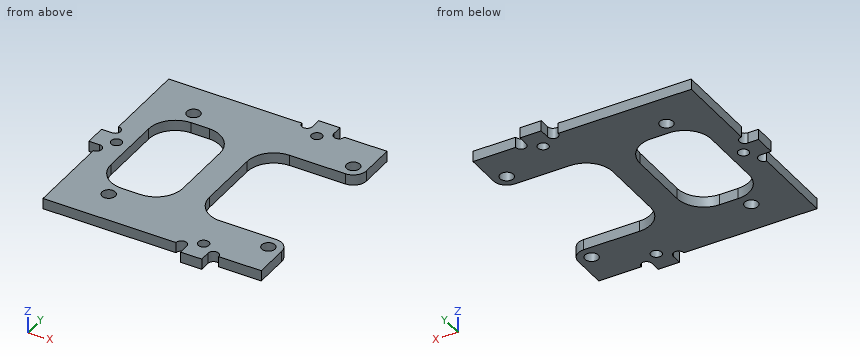
from build123d import *

# Parameters (mm, degrees)
SKETCH_1_R          = 1.25
SKETCH_1_R_2        = 1
EXTRUDE_1_DEPTH     = 2
SKETCH_4_W          = 18
SKETCH_4_H          = 22
CUT_EXTRUDE_1_DEPTH = 2
FILLET_2_R          = 2.5
FILLET_3_R          = 5
CUT_EXTRUDE_2_DEPTH = 2
SKETCH_7_R          = 1
CUT_EXTRUDE_3_DEPTH = 10
SKETCH_8_W          = 4
SKETCH_8_H          = 2
EXTRUDE_2_DEPTH     = 2
CUT_EXTRUDE_4_DEPTH = 2


with BuildPart() as part:
    # 草圖1 → 填料-伸長1 (new body)
    with BuildSketch(Plane.XY):
        Polygon((15.283786802, 18.1625), (-25.716213198, 18.1625), (-25.716213198, 0.1625), (-27.716213198, 0.1625), (-27.716213198, -3.8375), (-25.716213198, -3.8375), (-25.716213198, -21.8375), (15.283786802, -21.8375), align=None)
        with Locations((-17.216213198, 11.6625)):
            Circle(SKETCH_1_R, mode=Mode.SUBTRACT)
        with Locations((-17.216213198, -15.3375)):
            Circle(SKETCH_1_R, mode=Mode.SUBTRACT)
        with Locations((12.783786802, -15.3375)):
            Circle(SKETCH_1_R, mode=Mode.SUBTRACT)
        with Locations((12.783786802, 11.6625)):
            Circle(SKETCH_1_R, mode=Mode.SUBTRACT)
        with Locations((-23.716213198, -1.8375)):
            Circle(SKETCH_1_R_2, mode=Mode.SUBTRACT)
    extrude(amount=EXTRUDE_1_DEPTH)

    # 草圖4 → 除料-伸長1 (cut)
    with BuildSketch(Plane(origin=(0, 0, 0), x_dir=(-1, 0, 0), z_dir=(0, 0, -1))):
        with Locations((-6.283786802, -1.8375)):
            Rectangle(SKETCH_4_W, SKETCH_4_H)
    extrude(amount=-CUT_EXTRUDE_1_DEPTH, mode=Mode.SUBTRACT)

    # 圓角2
    fillet_2_edges = [part.edges().sort_by_distance(p)[0] for p in [
        (15.283786802, -12.8375, 1),
        (15.283786802, 9.1625, 1),
    ]]
    fillet(fillet_2_edges, radius=FILLET_2_R)

    # 圓角3
    fillet_3_edges = [part.edges().sort_by_distance(p)[0] for p in [
        (-2.716213198, 9.1625, 1),
        (-2.716213198, -12.8375, 1),
    ]]
    fillet(fillet_3_edges, radius=FILLET_3_R)

    # 草圖5 → 除料-伸長2 (cut)
    with BuildSketch(Plane(origin=(0, 0, 0), x_dir=(-1, 0, 0), z_dir=(0, 0, -1))):
        with BuildLine():
            Line((7.716213198, 3.948031945), (7.716213198, -7.8375))
            ThreePointArc((7.716213198, -7.8375), (9.180679292, -11.373033906), (12.716213198, -12.8375))
            Line((12.716213198, -12.8375), (16.216213198, -12.8375))
            ThreePointArc((16.216213198, -12.8375), (19.751747104, -11.373033906), (21.216213198, -7.8375))
            Line((21.216213198, -7.8375), (21.216213198, 4.1625))
            ThreePointArc((21.216213198, 4.1625), (19.751747104, 7.698033906), (16.216213198, 9.1625))
            Line((16.216213198, 9.1625), (12.716213198, 9.1625))
            ThreePointArc((12.716213198, 9.1625), (9.168164983, 7.56020857), (7.716213198, 3.948031945))
        make_face()
    extrude(amount=-CUT_EXTRUDE_2_DEPTH, mode=Mode.SUBTRACT)

    # 草圖7 → 除料-伸長3 (cut)
    with BuildSketch(Plane(origin=(0, 0, 0), x_dir=(-1, 0, 0), z_dir=(0, 0, -1))):
        with Locations((-3.283786802, -19.8375)):
            Circle(SKETCH_7_R)
        with Locations((-3.283786802, 16.1625)):
            Circle(SKETCH_7_R)
    extrude(amount=-CUT_EXTRUDE_3_DEPTH, mode=Mode.SUBTRACT)

    # 草圖8 → 填料-伸長2 (add)
    with BuildSketch(Plane(origin=(0, 0, 0), x_dir=(-1, 0, 0), z_dir=(0, 0, -1))):
        with Locations((-3.283786802, 19.1625)):
            Rectangle(SKETCH_8_W, SKETCH_8_H)
        with Locations((-3.283786802, -22.8375)):
            Rectangle(SKETCH_8_W, SKETCH_8_H)
    extrude(amount=-EXTRUDE_2_DEPTH)

    # 草圖9 → 除料-伸長4 (cut)
    with BuildSketch(Plane(origin=(0, 0, 0), x_dir=(-1, 0, 0), z_dir=(0, 0, -1))):
        with BuildLine():
            Line((-7.283786802, 18.1625), (-5.283786802, 18.1625))
            ThreePointArc((-5.283786802, 18.1625), (-6.283786802, 17.1625), (-7.283786802, 18.1625))
        make_face()
        with BuildLine():
            Line((-1.283786802, 18.1625), (0.716213198, 18.1625))
            ThreePointArc((0.716213198, 18.1625), (-0.283786802, 17.1625), (-1.283786802, 18.1625))
        make_face()
        with BuildLine():
            Line((-7.283786802, -21.8375), (-5.283786802, -21.8375))
            ThreePointArc((-5.283786802, -21.8375), (-6.283786802, -20.8375), (-7.283786802, -21.8375))
        make_face()
        with BuildLine():
            Line((-1.283786802, -21.8375), (0.716213198, -21.8375))
            ThreePointArc((0.716213198, -21.8375), (-0.283786802, -20.8375), (-1.283786802, -21.8375))
        make_face()
        with BuildLine():
            Line((25.716213198, 2.1625), (25.716213198, 0.1625))
            ThreePointArc((25.716213198, 0.1625), (24.716213198, 1.1625), (25.716213198, 2.1625))
        make_face()
        with BuildLine():
            Line((25.716213198, -3.8375), (25.716213198, -5.8375))
            ThreePointArc((25.716213198, -5.8375), (24.716213198, -4.8375), (25.716213198, -3.8375))
        make_face()
    extrude(amount=-CUT_EXTRUDE_4_DEPTH, mode=Mode.SUBTRACT)


solid = part.part
Here's how the part is built. I have some questions about the finished solid (model axes, mm). Give positions to 0.01 mm unless a question says otherwise; leave off trailing zeros. Loops run counter-clockwise (first coordinate to the right, second up) from the corner with the lowest first, then second, coordinate; pieces in that order, holes last. Notation, with made-up numbers: (-33.75, 47.25) -> (-29.75, 47.25) arc R23 ccw to (-29.75, 69.25) -> close; hole circle Ø9 at (76, 33.25). An arc over 180 degrees is marked (long way). Answer as a JSON object with one key per item and string values. Group by question number.
Item 1: Will these pins go through, and if not, where does the flat tip stop? pin 1 (1.2 mm diameter, centred on x = -23.72, y = -1.84, fed in from +Z); pin 2 (3 mm diameter, centred on x = -17.22, y = 11.66, fed in from +Z); pin 3 (1 mm diameter, centred on y = 13, z = 1.5, fed in from -X); pin 4 (1 mm diameter, centred on x = 7, z = 1, fed in from -Y).
Item 2: Imagine slicing it at C-C on x = 3. Write out the boundary of the cut face in (y, z).
Item 3: Imagine slicing it at A-A on x = 8.5. Write out the boundary of the cut face in (y, z), then the cut area to 3 significant figures.
Item 4: Imagine slicing it at B-B on y = -10. Write out the boundary of the cut face in (x, z).
Item 5: Imagine slicing it at D-D on z = 0.9. Give the number of separate pieces and of enclosed holes in the cut face, then the cut area to 3 significant figures.
Item 6: I need wall thicknesses on L1, parallel to Y at x = 4.5, z = 0.2; L2, parallel to Y at x = 8.5, z = 1.9; L3, parallel to X at y = -6.5, z = 1.8. Which ranges of each line are inside material? Lowest first, please.
Answer list:
{
 "1": {"pin 1": "passes through", "pin 2": "stops at z = 2", "pin 3": "stops at x = -25.72", "pin 4": "stops at y = -21.84"},
 "2": {"outline": "(-23.84, 0) -> (-20.8, 0) -> (-20.8, 2) -> (-23.84, 2) -> close; (-18.88, 0) -> (-12.84, 0) -> (-12.84, 2) -> (-18.88, 2) -> close; (9.16, 0) -> (15.2, 0) -> (15.2, 2) -> (9.16, 2) -> close; (17.12, 0) -> (20.16, 0) -> (20.16, 2) -> (17.12, 2) -> close"},
 "3": {"outline": "(-21.84, 0) -> (-12.84, 0) -> (-12.84, 2) -> (-21.84, 2) -> close; (9.16, 0) -> (18.16, 0) -> (18.16, 2) -> (9.16, 2) -> close", "area": "36.0 mm2"},
 "4": {"outline": "(-25.72, 0) -> (-20.72, 0) -> (-20.72, 2) -> (-25.72, 2) -> close; (-8.21, 0) -> (-2.22, 0) -> (-2.22, 2) -> (-8.21, 2) -> close"},
 "5": {"separate pieces": "1", "enclosed holes": "8", "area": "962 mm2"},
 "6": {"L1": "y = -23.84 to -12.84, 9.16 to 20.16", "L2": "y = -21.84 to -12.84, 9.16 to 18.16", "L3": "x = -25.72 to -21.22, -7.72 to -2.72"}
}
